Part model, mm, in its own coordinate system. Face numbers are marked on the shaded views. A direction names the side the tool comes from. Coordinates: 2 decimals unless noted, no trailing zeros. Loops run counter-clockwise (first coordinate to the right, second up) from the corner with the lowest first, then second, coordinate; pieces in that order, holes last. Notation, with made-up numbers: (53.5, -33) -> (110.5, -33) arc R16 ccw to (110.5, -10) -> close; hole circle Ø9 at (14.5, -20). An arc over 180 degrees is marked (long way). Use one line per item in the form item = value. Start each with the question number.
(1) 3-axis set-ups, long thin cutter, end or side, ignore diameter. For the marked faces 3 and 4: which of +Z, -Z, +X, -X, +Y, -Y reach the whole face in a straight line?
(2) Drill centre lines: L1, parallel to Y at x = 140.3, z = 2; L2, parallel to X at y = 19.5, z = -13; L3, parallel to Z at x = -38, y = 51.5. Where is each one in solid material? Low to high. Write a range as [from, to].
(3) Band-saw the part on A-A on z = -21.5. Give the cut face in (x, y), then the cut area to 3 significant figures.
(4) Mould opens along Z. For the marked faces 1 and 2 say: +Z half, -Z half, draft (parallel to the pull), parting line (faces both ways), or undercut.
(5) Band-saw the part on D-D on x = 34.5. Give the cut face in (y, z).
(6) Band-saw the part on C-C on x = 140.3. Give the cut face in (y, z).
(7) Band-saw the part on B-B on y = 57.4. Give the cut face in (x, z), then the cut area to 3 significant figures.
(8) Pin check, flat tips, straight feed: P1, Ø10, axis at x = 212, z = -13, coming from the +Y side; P2, Ø12.5, axis at x = 188, z = -12.5, coming from the -Y side; P3, Ø1.8, axis at y = 8.5, z = -17, coming from the +X side; P4, Ø5, axis at x = 50, z = -4.5, coming from the -Y side. Stop position of each tip, or through.
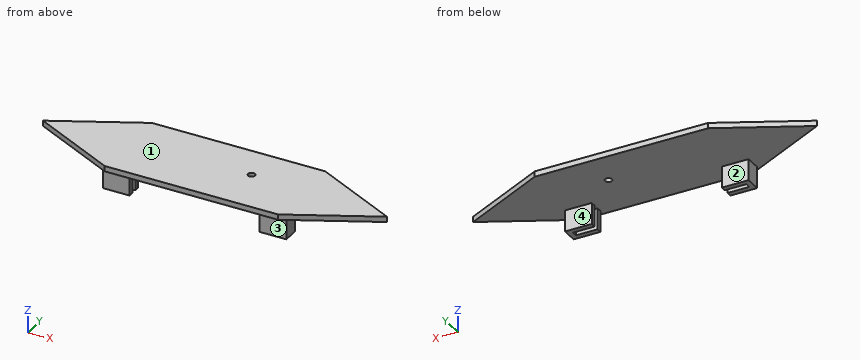
```python
from build123d import *

# Parameters (mm, degrees)
BOSS_EXTRUDE1_DEPTH = 6.35
BOSS_EXTRUDE3_DEPTH = 25
SKETCH3_R           = 4
CUT_EXTRUDE1_DEPTH  = 25


with BuildPart() as part:
    # Sketch1 → Boss-Extrude1 (new body)
    with BuildSketch(Plane.XY):
        Polygon((0, 0), (203.2, 0), (303.2, 50), (203.2, 100), (0, 100), (-100, 50), align=None)
    extrude(amount=BOSS_EXTRUDE1_DEPTH)

    # Sketch2 → Boss-Extrude3 (add)
    with BuildSketch(Plane(origin=(0, 0, 0), x_dir=(-1, 0, 0), z_dir=(0, 0, -1))):
        Polygon((-177.8, 12.7), (-203.2, 12.7), (-203.2, 19.05), (-177.8, 19.05), (-177.8, 25.05), (-209.2, 25.05), (-209.2, 6.7), (-177.8, 6.7), align=None)
        Polygon((6, 6.7), (6, 25.05), (-25.4, 25.05), (-25.4, 19.05), (0, 19.05), (0, 12.7), (-25.4, 12.7), (-25.4, 6.7), align=None)
    extrude(amount=BOSS_EXTRUDE3_DEPTH)

    # Sketch3 → Cut-Extrude1 (cut)
    with BuildSketch(Plane(origin=(0, 0, 0), x_dir=(-1, 0, 0), z_dir=(0, 0, -1))):
        with Locations((-140.3, 57.4)):
            Circle(SKETCH3_R)
    extrude(amount=-CUT_EXTRUDE1_DEPTH, mode=Mode.SUBTRACT)


solid = part.part
```
A:
q1.face_3 = -Z, +X, -X, -Y
q1.face_4 = -Z, +X, -X, +Y
q2.L1 = [0, 53.4], [61.4, 100]
q2.L2 = [-6, 25.4], [177.8, 209.2]
q2.L3 = [0, 6.35]
q3.outline = (-6, 6.7) -> (25.4, 6.7) -> (25.4, 12.7) -> (0, 12.7) -> (0, 19.05) -> (25.4, 19.05) -> (25.4, 25.05) -> (-6, 25.05) -> close; (177.8, 6.7) -> (209.2, 6.7) -> (209.2, 25.05) -> (177.8, 25.05) -> (177.8, 19.05) -> (203.2, 19.05) -> (203.2, 12.7) -> (177.8, 12.7) -> close
q3.area = 830 mm²
q4.face_1 = +Z half
q4.face_2 = draft
q5.outline = (0, 0) -> (100, 0) -> (100, 6.35) -> (0, 6.35) -> close
q6.outline = (0, 0) -> (53.4, 0) -> (53.4, 6.35) -> (0, 6.35) -> close; (61.4, 0) -> (100, 0) -> (100, 6.35) -> (61.4, 6.35) -> close
q7.outline = (-85.2, 0) -> (136.3, 0) -> (136.3, 6.35) -> (-85.2, 6.35) -> close; (144.3, 0) -> (288.4, 0) -> (288.4, 6.35) -> (144.3, 6.35) -> close
q7.area = 2,320 mm²
q8.P1 = 25.05
q8.P2 = 6.7
q8.P3 = 209.2
q8.P4 = through
